Could you check a few things on this model? Use its own coordinates, in mm. A direction names the side the tool comes from. Give positions to 0.01 mm unless a question says otherwise; leave off trailing zeros. Write each loop counter-clockwise with the first axis right and the second up, starting at its lowest first coordinate (ties: lowest second). Pieces come first, ordered by that corner, then holes. Notation, with made-up numbers: (52, 60.25) - (62, 60.25) arc R25 ccw to (62, 81.25) - close; hole circle Ø6 at (42.5, 21). An arc over 180 degrees is marked (long way). Use one line per item in the form item = value.
```python
from build123d import *

# Parameters (mm, degrees)
SKETCH1_R           = 26
BOSS_EXTRUDE1_DEPTH = 6
SKETCH1_4_R         = 3
BOSS_EXTRUDE2_DEPTH = 0.6


with BuildPart() as part:
    # Sketch1 → Boss-Extrude1 (new body)
    with BuildSketch(Plane(origin=(0, 0, 0), x_dir=(1, 0, 0), z_dir=(0, 1, 0))):
        with Locations(Location((0, 0, 0), (0, 0, 270))):
            Circle(SKETCH1_R)
        with BuildLine():
            ThreePointArc((-4.433155886, 0.772741152), (-4.279754323, -1.390576475), (-3.132292598, -3.230904375))
            Line((-3.132292598, -3.230904375), (-15.722136801, -15.388775598))
            ThreePointArc((-15.722136801, -15.388775598), (-20.923243358, -6.798373876), (-21.764771207, 3.208540836))
            Line((-21.764771207, 3.208540836), (-4.433155886, 0.772741152))
        make_face(mode=Mode.SUBTRACT)
        with BuildLine():
            ThreePointArc((-2.104841015, -3.977391645), (0, -4.5), (2.104841015, -3.977391645))
            Line((2.104841015, -3.977391645), (9.777187851, -19.708033837))
            ThreePointArc((9.777187851, -19.708033837), (0, -22), (-9.777187851, -19.708033837))
            Line((-9.777187851, -19.708033837), (-2.104841015, -3.977391645))
        make_face(mode=Mode.SUBTRACT)
        with BuildLine():
            ThreePointArc((3.132292598, -3.230904375), (4.279754323, -1.390576475), (4.433155886, 0.772741152))
            Line((4.433155886, 0.772741152), (21.764771207, 3.208540836))
            ThreePointArc((21.764771207, 3.208540836), (20.923243358, -6.798373876), (15.722136801, -15.388775598))
            Line((15.722136801, -15.388775598), (3.132292598, -3.230904375))
        make_face(mode=Mode.SUBTRACT)
        with BuildLine():
            Line((-2.928736929, 0.65), (2.928736929, 0.65))
            ThreePointArc((2.928736929, 0.65), (0, -3), (-2.928736929, 0.65))
        make_face(mode=Mode.SUBTRACT)
        with BuildLine():
            ThreePointArc((-0.635, 4.454971942), (-2.645033635, 3.640576475), (-4.040704303, 1.980582927))
            Line((-4.040704303, 1.980582927), (-19.49400277, 10.197247472))
            ThreePointArc((-19.49400277, 10.197247472), (-12.93127555, 17.798373876), (-3.674180512, 21.691021128))
            Line((-3.674180512, 21.691021128), (-0.635, 4.454971942))
        make_face(mode=Mode.SUBTRACT)
        with BuildLine():
            Line((0.635, 4.454971942), (3.674180512, 21.691021128))
            ThreePointArc((3.674180512, 21.691021128), (12.93127555, 17.798373876), (19.49400277, 10.197247472))
            Line((19.49400277, 10.197247472), (4.040704303, 1.980582927))
            ThreePointArc((4.040704303, 1.980582927), (2.645033635, 3.640576475), (0.635, 4.454971942))
        make_face(mode=Mode.SUBTRACT)
    extrude(amount=BOSS_EXTRUDE1_DEPTH)

    # Sketch1_4 → Boss-Extrude2 (add)
    with BuildSketch(Plane(origin=(0, 0, 0), x_dir=(1, 0, 0), z_dir=(0, 1, 0))):
        Circle(SKETCH1_4_R)
    extrude(amount=BOSS_EXTRUDE2_DEPTH)


solid = part.part
```
1. If I drill on line 1 (X direction, y = 4.45, z = 0); line 2 (X direction, y = 3.9, z = -4); line 3 (X direction, y = 2.6, z = 8), over which ranges is the centre line in solid material (lowest first)? Write a range as from..to.
Response values:
line_1 = -26..-22, -4.5..-3, 3..4.5, 22..26
line_2 = -25.69..-7.84, -2.06..2.06, 7.84..25.69
line_3 = -24.74..-20.49, -8.07..-4.07, 4.07..8.07, 20.49..24.74
2. Imagine slicing it at B-B, the plane z = 0. List the corners of the cut face in (x, y) for me, and give its area (3 significant figures).
Response values:
outline = (-26, 0) - (-22, 0) - (-22, 6) - (-26, 6) - close; (-4.5, 0) - (4.5, 0) - (4.5, 6) - (3, 6) - (3, 0.6) - (-3, 0.6) - (-3, 6) - (-4.5, 6) - close; (22, 0) - (26, 0) - (26, 6) - (22, 6) - close
area = 69.6 mm²
3. Which directions (+Z, -Z, +X, -X, +Y, -Y) give clear straight access to the entire face, cutting with the end or side of a thin tool? Please do faces 3 (the face through (0, 3, 3)), 4 (the face through (0, 6, -6)), 5 (the face through (0, 3, 4.5)).
Response values:
face_3 = +Y
face_4 = +Z, -Z, +X, -X, +Y
face_5 = +Y, -Y
4. Imagine slicing it at D-D, the plane x = -18.5. List the corners of the cut face in (y, z) for me.
Response values:
outline = (0, -18.27) - (6, -18.27) - (6, -11.91) - (0, -11.91) - close; (0, -9.67) - (6, -9.67) - (6, -2.75) - (0, -2.75) - close; (0, 11.91) - (6, 11.91) - (6, 18.27) - (0, 18.27) - close
5. If we mould it in two halves opening along Z, with no side actions, what happens to faces 1 (the face through (-5.995, 2.958, 11.953)), 2 (the face through (0, 0, 0))? For each: pulls with the +Z half, pulls with the -Z half, needs draft (parallel to the pull), parting line crosses it, or undercut.
Response values:
face_1 = undercut
face_2 = needs draft
6. For pin 1 (3 mm diameter, centred on x = 18.5, y = 3, fed in from +Z); pin 2 (1 mm diameter, centred on y = 5, z = -11.5, fed in from -X); pin 3 (1 mm diameter, centred on y = 1.5, z = 16.5, fed in from -X), each with a flat end and sliding along its axis, tell me the tip position at first contact or that it passes through.
Response values:
pin_1 = 19.67
pin_2 = -23.56
pin_3 = -20.49
7. Imagine slicing it at C-C, the plane y = 5.2. List the corners of the cut face in (x, z) for me (3 decimals), and give its area (3 significant figures).
Response values:
outline = circle Ø52 at (0, 0); hole (-21.765, -3.209) - (-4.433, -0.773) arc R4.5 cw to (-3.132, 3.231) - (-15.722, 15.389) arc R22 ccw to start; hole (-19.494, -10.197) arc R22 ccw to (-3.674, -21.691) - (-0.635, -4.455) arc R4.5 cw to (-4.041, -1.981) - close; hole (-9.777, 19.708) - (-2.105, 3.977) arc R4.5 cw to (2.105, 3.977) - (9.777, 19.708) arc R22 ccw to start; hole (-2.929, -0.65) - (2.929, -0.65) arc R3 ccw (long way) to start; hole (0.635, -4.455) - (3.674, -21.691) arc R22 ccw to (19.494, -10.197) - (4.041, -1.981) arc R4.5 cw to start; hole (3.132, 3.231) arc R4.5 cw to (4.433, -0.773) - (21.765, -3.209) arc R22 ccw to (15.722, 15.389) - close
area = 1,030 mm²
8. Imagine slicing it at A-A, the plane x = 0. List the corners of the cut face in (y, z) for me, and give its area (3 significant figures).
Response values:
outline = (0, -26) - (6, -26) - (6, -0.65) - (0.6, -0.65) - (0.6, 3) - (6, 3) - (6, 4.5) - (0, 4.5) - close; (0, 22) - (6, 22) - (6, 26) - (0, 26) - close
area = 187 mm²
